Geometry: final body of the model. Coordinates: model frame, mm. Round coordinates to 2 decimals unless told otherwise and drop trailing zeros. Write each loop counter-clockwise with the first axis right and the second up, starting at its lowest first coordinate (ties: lowest second). Pieces come first, ordered by that corner, then holes. Notation, with made-up numbers: M 26.5,64 L 55.5,64 A24 ccw 55.5,84 Z; hole C 72,-23 d8. An arc over 180 degrees is marked long. Use one line per item in the form item = value. Start each with the question number.
Item 1: Section query C-C (x = 140). Return loops of the section in (y, z).
Item 2: Section query B-B (x = 109). Return loops of the section in (y, z), and give its area (3 significant figures).
Item 3: Section query A-A (y = 88.5). Return loops of the section in (x, z).
Item 4: Ray query, probe 1 along Y at (x, z) = (140, 2.55); probe 2 along Y at (x, z) = (119.5, 2.3); probe 3 along X at (y, z) = (33, 1.05). Return the intervals inside material, ascending.
Item 5: Section query D-D (z = 1.95). State how many separate pieces and enclosed holes the cut face has, and give its area (3 significant figures).
from build123d import *

# Parameters (mm, degrees)
CYLINDER004_R     = 1.8
CYLINDER004_DEPTH = 20
ARRAY007_X_COUNT  = 2
ARRAY007_X_PITCH  = 81
ARRAY007_Y_COUNT  = 2
ARRAY007_Y_PITCH  = 55.5
CYLINDER003_R     = 1.8
CYLINDER003_DEPTH = 30
ARRAY004_X_COUNT  = 4
ARRAY004_X_PITCH  = 57.666667
ARRAY005_Y_COUNT  = 2
ARRAY005_Y_PITCH  = 114.4
ARRAY002_Y_COUNT  = 4
ARRAY002_Y_PITCH  = 38.133333
ARRAY003_X_COUNT  = 2
ARRAY003_X_PITCH  = 173
BOX019_W          = 40
BOX019_H          = 8
BOX019_DEPTH      = 10
BOX018_W          = 181
BOX018_H          = 122.4
BOX018_DEPTH      = 3.3
FILLET001_R       = 3


with BuildPart() as array007:
    # Cylinder004 → Cylinder004 (new body)
    with BuildSketch(Plane(origin=(59, 33, -7), x_dir=(1, 0, 0), z_dir=(0, 0, 1))):
        Circle(CYLINDER004_R)
    extrude(amount=CYLINDER004_DEPTH)

    # Array007 X: Array007 ×2


with BuildPart() as array007_1:
    add(array007.part)
    with Locations(*[(i * ARRAY007_X_PITCH, 0, 0) for i in range(1, ARRAY007_X_COUNT)]):
        add(array007.part)

    # Array007 Y: Array007 ×2


with BuildPart() as array007_2:
    add(array007_1.part)
    with Locations(*[(0, i * ARRAY007_Y_PITCH, 0) for i in range(1, ARRAY007_Y_COUNT)]):
        add(array007_1.part)


with BuildPart() as cylinder003:
    # Cylinder003 → Cylinder003 (new body)
    with BuildSketch(Plane(origin=(4, 4, 1), x_dir=(1, 0, 0), z_dir=(0, 0, 1))):
        Circle(CYLINDER003_R)
    extrude(amount=CYLINDER003_DEPTH)


with BuildPart() as array005:
    # Array004 base: copy of Cylinder003
    add(cylinder003.part)

    # Array004 X: Array005 ×4


with BuildPart() as array005_1:
    add(array005.part)
    with Locations(*[(i * ARRAY004_X_PITCH, 0, 0) for i in range(1, ARRAY004_X_COUNT)]):
        add(array005.part)

    # Array005 Y: Array005 ×2


with BuildPart() as array005_2:
    add(array005_1.part)
    with Locations(*[(0, i * ARRAY005_Y_PITCH, 0) for i in range(1, ARRAY005_Y_COUNT)]):
        add(array005_1.part)


with BuildPart() as side_wider_holes_clone:
    # Array002 base: copy of Cylinder003
    add(cylinder003.part)

    # Array002 Y: side wider holes clone ×4


with BuildPart() as side_wider_holes_clone_1:
    add(side_wider_holes_clone.part)
    with Locations(*[(0, i * ARRAY002_Y_PITCH, 0) for i in range(1, ARRAY002_Y_COUNT)]):
        add(side_wider_holes_clone.part)

    # Array003 X: side wider holes clone ×2


with BuildPart() as side_wider_holes_clone_2:
    add(side_wider_holes_clone_1.part)
    with Locations(*[(i * ARRAY003_X_PITCH, 0, 0) for i in range(1, ARRAY003_X_COUNT)]):
        add(side_wider_holes_clone_1.part)

    # Fusion009: union Array005
    add(array005_2.part)


with BuildPart() as side_wider_holes_clone_3:
    # Body024 placement: moved
    add(side_wider_holes_clone_2.part.moved(Location((0, 0, -8))))


with BuildPart() as fusion006:
    # Box019 → Box019 (new body)
    with BuildSketch(Plane(origin=(71, 6, -2), x_dir=(1, 0, 0), z_dir=(0, 0, 1))):
        with Locations((20, 4)):
            Rectangle(BOX019_W, BOX019_H)
    extrude(amount=BOX019_DEPTH)

    # Fusion006: union Array007, side wider holes clone
    add(array007_2.part)
    add(side_wider_holes_clone_3.part)


with BuildPart() as display_back_cut:
    # Box018 → Box018 (new body)
    with BuildSketch(Plane.XY):
        with Locations((90.5, 61.2)):
            Rectangle(BOX018_W, BOX018_H)
    extrude(amount=BOX018_DEPTH)

    # Fillet001
    fillet001_edges = [display_back_cut.edges().sort_by_distance(p)[0] for p in [
        (0, 0, 1.65),
        (0, 122.4, 1.65),
        (181, 0, 1.65),
        (181, 122.4, 1.65),
    ]]
    fillet(fillet001_edges, radius=FILLET001_R)

    # Cut003: cut Fusion006
    add(fusion006.part, mode=Mode.SUBTRACT)


solid = display_back_cut.part
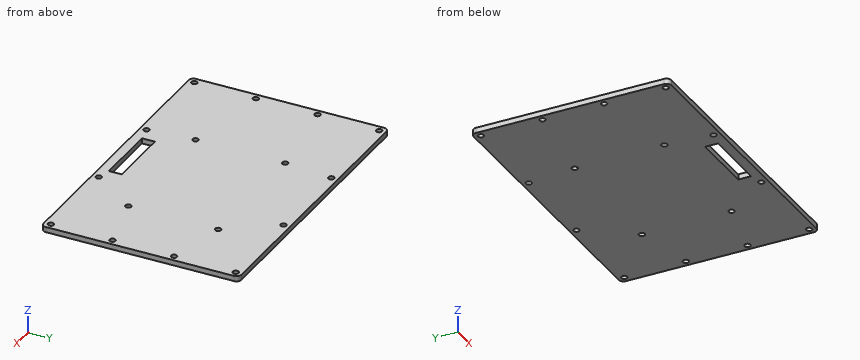
Working result:
q1.outline = M 0,0 L 31.2,0 L 31.2,3.3 L 0,3.3 Z; M 34.8,0 L 86.7,0 L 86.7,3.3 L 34.8,3.3 Z; M 90.3,0 L 122.4,0 L 122.4,3.3 L 90.3,3.3 Z
q2.outline = M 0,0 L 6,0 L 6,3.3 L 0,3.3 Z; M 14,0 L 122.4,0 L 122.4,3.3 L 14,3.3 Z
q2.area = 378 mm²
q3.outline = M 0,0 L 57.2,0 L 57.2,3.3 L 0,3.3 Z; M 60.8,0 L 138.2,0 L 138.2,3.3 L 60.8,3.3 Z; M 141.8,0 L 181,0 L 181,3.3 L 141.8,3.3 Z
q4.probe_1 = 0 to 31.2, 34.8 to 86.7, 90.3 to 122.4
q4.probe_2 = 0 to 2.21, 5.79 to 116.61, 120.19 to 122.4
q4.probe_3 = 0 to 57.2, 60.8 to 138.2, 141.8 to 181
q5.separate_pieces = 1
q5.enclosed_holes = 17
q5.area = 21,700 mm²
